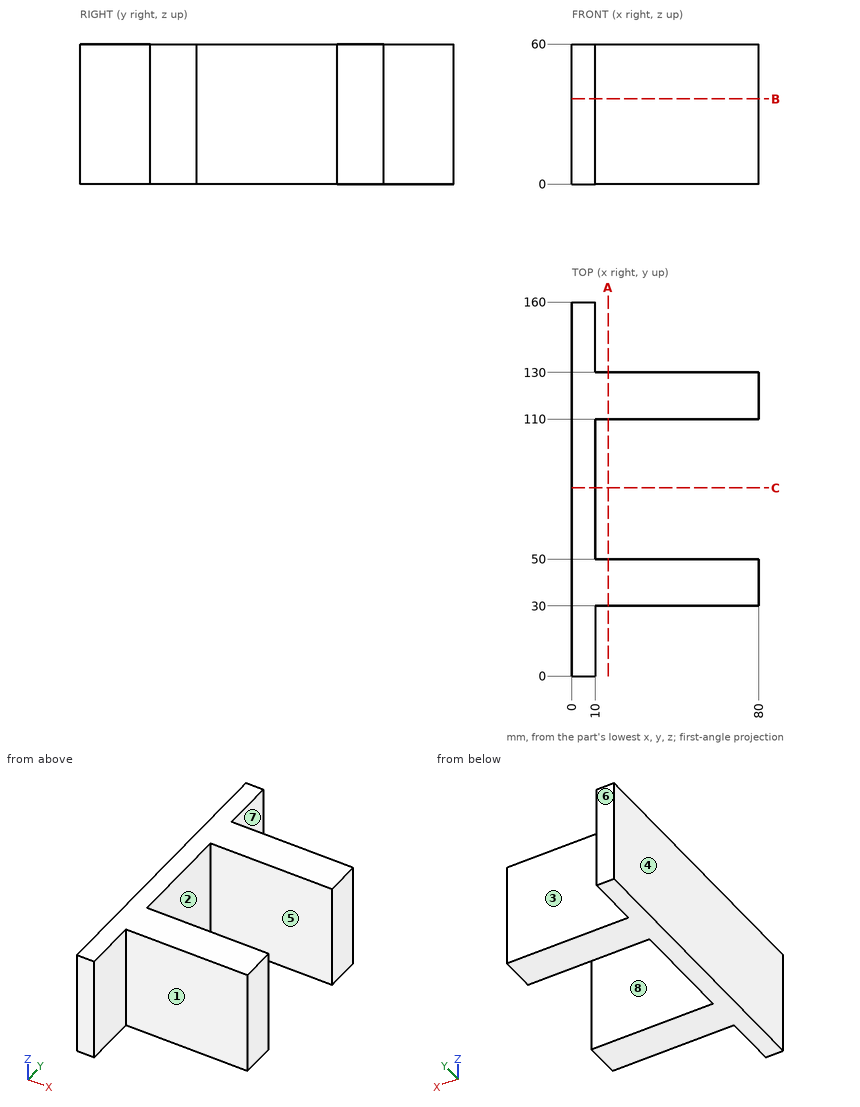
For this review, use the dimensioned drawing (mm, ordinates from the lowest corner) and the shaded views. A direction names the side the tool comes from. Give positions to 0.01 mm unless a question says otherwise; leave off trailing zeros. Order: outer loops, then holes, each group sorted by start corner. A loop starts at its lowest first (then second) coordinate and runs counter-clockwise, first axis right, second up.
1. Tool access review of the marked faces 1, 2, 3 and 4: name each direction out of +Z, -Z, +X, -X, +Y, -Y from which nothing blocks a thin tool from reaching the whole face with its end or side.
Solution:
face 1: +Z, -Z, +X, -Y
face 2: +Z, -Z, +X
face 3: +Z, -Z, +X, +Y
face 4: +Z, -Z, -X, +Y, -Y
2. Mouldability with a two-part tool opening along Y and no side actions: class the marked faces 5, 6, 7 and 8 as +Y half, -Y half, draft (parallel to the pull), parting line (faces both ways), or undercut.
Solution:
face 5: undercut
face 6: +Y half
face 7: draft
face 8: undercut
3. To check wall thickness, follow L1, parallel to Y at x = 30.5, z = 3.5; L2, parallel to X at y = 152.5, z = 28.5. State the ranges of each line that lie inside material, in increasing order.
Solution:
L1: y = 30 to 50, 110 to 130
L2: x = 0 to 10
4. Add section C-C, the plane y = 80.5. State the section outline as (x, z) points.
Solution:
outline: (0, 0) - (10, 0) - (10, 60) - (0, 60) - close
5. For pin 1 Ø10 at (y, z) = (76.5, 32) entering from +X; pin 2 Ø4 at (x, z) = (18.5, 6.5) entering from -Y; pin 3 Ø1.5 at (x, z) = (20.5, 17) entering from +Y, all flat-tipped, find the tip position at first contact; note any pin that passes through.
Solution:
pin 1: stops at x = 10
pin 2: stops at y = 30
pin 3: stops at y = 130
6. Add section A-A, the plane x = 15.5. State the section outline as (y, z) points.
Solution:
outline: (30, 0) - (50, 0) - (50, 60) - (30, 60) - close; (110, 0) - (130, 0) - (130, 60) - (110, 60) - close
7. Add section B-B, the plane z = 36.5. State the section outline as (x, y) points, then the cut area to 3 significant figures.
Solution:
outline: (0, 0) - (10, 0) - (10, 30) - (80, 30) - (80, 50) - (10, 50) - (10, 110) - (80, 110) - (80, 130) - (10, 130) - (10, 160) - (0, 160) - close
area: 4,400 mm2
